from build123d import *

# Parameters (mm, degrees)
BOSS_EXTRUDE1_DEPTH            = 25
CUT_EXTRUDE1_REACH             = 60.44
SKETCH2_R                      = 2.25
SKETCH3_W                      = 25
SKETCH3_H                      = 63
SKETCH3_R                      = 3.75
BOSS_EXTRUDE2_DEPTH            = 2
FILLET1_R                      = 3
SKETCH4_R                      = 2.55
CUT_EXTRUDE2_DEPTH             = 3.5
SKETCH4_3_R                    = 2.55
CUT_EXTRUDE5_DEPTH             = 6.5
SKETCH6_W                      = 10
SKETCH6_H                      = 1.25
SKETCH5_R                      = 1.5
CUT_EXTRUDE3_DEPTH             = 1
SKETCH5_2_R                    = 1.5
CUT_EXTRUDE4_DEPTH             = 3.75
CUT_EXTRUDE4_DIRECTION_2_REACH = 59.567
CUT_EXTRUDE6_DEPTH             = 10


with BuildPart() as part:
    # Sketch1 → Boss-Extrude1 (new body)
    with BuildSketch(Plane(origin=(0, 0, 0), x_dir=(0, 0, -1), z_dir=(1, 0, 0))):
        Polygon((8.75, 0), (8.75, 9.25), (9.5, 10), (15.25, 10), (15.25, 23), (-19.25, 23), (-19.25, -40), (-16.25, -40), (-16.25, 0), (-12.5, 0), (-12.5, 8.25), (0, 8.25), (0, 0), (3.75, 0), align=None)
    extrude(amount=BOSS_EXTRUDE1_DEPTH)

    # Sketch2 → Cut-Extrude1 (cut, up to next)
    with BuildSketch(Plane.XY.offset(19.25), mode=Mode.PRIVATE) as cut_extrude1_sk1:
        with Locations((6.25, -30)):
            Circle(SKETCH2_R)
    cut_extrude1_tool1 = extrude(cut_extrude1_sk1.sketch, amount=-CUT_EXTRUDE1_REACH, mode=Mode.PRIVATE) & part.part
    # Sketch2 → Cut-Extrude1 (cut, up to next)
    with BuildSketch(Plane.XY.offset(19.25), mode=Mode.PRIVATE) as cut_extrude1_sk2:
        with Locations((6.25, -10)):
            Circle(SKETCH2_R)
    cut_extrude1_tool2 = extrude(cut_extrude1_sk2.sketch, amount=-CUT_EXTRUDE1_REACH, mode=Mode.PRIVATE) & part.part
    # Sketch2 → Cut-Extrude1 (cut, up to next)
    with BuildSketch(Plane.XY.offset(19.25), mode=Mode.PRIVATE) as cut_extrude1_sk3:
        with Locations((6.25, 16)):
            Circle(SKETCH2_R)
    cut_extrude1_tool3 = extrude(cut_extrude1_sk3.sketch, amount=-CUT_EXTRUDE1_REACH, mode=Mode.PRIVATE) & part.part
    # Sketch2 → Cut-Extrude1 (cut, up to next)
    with BuildSketch(Plane.XY.offset(19.25), mode=Mode.PRIVATE) as cut_extrude1_sk4:
        with Locations((19, 16)):
            Circle(SKETCH2_R)
    cut_extrude1_tool4 = extrude(cut_extrude1_sk4.sketch, amount=-CUT_EXTRUDE1_REACH, mode=Mode.PRIVATE) & part.part
    add(cut_extrude1_tool1.solids().sort_by_distance((6.25, -30, 19.25))[0], mode=Mode.SUBTRACT)
    add(cut_extrude1_tool2.solids().sort_by_distance((6.25, -10, 19.25))[0], mode=Mode.SUBTRACT)
    add(cut_extrude1_tool3.solids().sort_by_distance((6.25, 16, 19.25))[0], mode=Mode.SUBTRACT)
    add(cut_extrude1_tool4.solids().sort_by_distance((19, 16, 19.25))[0], mode=Mode.SUBTRACT)

    # Sketch3 → Boss-Extrude2 (add)
    with BuildSketch(Plane.XY.offset(19.25)):
        with Locations((12.5, -8.5)):
            Rectangle(SKETCH3_W, SKETCH3_H)
        with Locations((6.25, -30)):
            Circle(SKETCH3_R, mode=Mode.SUBTRACT)
        with Locations((6.25, -10)):
            Circle(SKETCH3_R, mode=Mode.SUBTRACT)
        Polygon((10, 18.165063509), (6.25, 20.330127019), (2.5, 18.165063509), (2.5, 13.834936491), (6.25, 11.669872981), (10, 13.834936491), align=None, mode=Mode.SUBTRACT)
        Polygon((19, 20.330127019), (15.25, 18.165063509), (15.25, 13.834936491), (19, 11.669872981), (22.75, 13.834936491), (22.75, 18.165063509), align=None, mode=Mode.SUBTRACT)
    extrude(amount=BOSS_EXTRUDE2_DEPTH)

    # Fillet1
    # the kernel refuses this fillet: 3 mm, written as the material it takes off along each edge
    with BuildSketch(Plane(origin=(3, 20, 18.25), x_dir=(0, 0, 1), z_dir=(-1, 0, 0))) as fillet1_piece_1_section:
        Polygon((0, 0), (FILLET1_R, 0), (FILLET1_R, FILLET1_R), (0, FILLET1_R), align=None)
    fillet1_piece_1 = extrude(amount=FILLET1_R, mode=Mode.PRIVATE)
    fillet1_piece_1 = fillet1_piece_1 - Plane(origin=(3, 20, 18.25), x_dir=(0, -0.7071067811865475, -0.7071067811865475), z_dir=(-1, 0, 0)) * Sphere(FILLET1_R, mode=Mode.PRIVATE)
    add(fillet1_piece_1, mode=Mode.SUBTRACT)
    with BuildSketch(Plane(origin=(22, 20, 18.25), x_dir=(0, 0, 1), z_dir=(1, 0, 0))) as fillet1_piece_2_section:
        Polygon((0, 0), (FILLET1_R, 0), (FILLET1_R, -FILLET1_R), (0, -FILLET1_R), align=None)
    fillet1_piece_2 = extrude(amount=FILLET1_R, mode=Mode.PRIVATE)
    fillet1_piece_2 = fillet1_piece_2 - Plane(origin=(22, 20, 18.25), x_dir=(0, -0.7071067811865475, -0.7071067811865475), z_dir=(1, 0, 0)) * Sphere(FILLET1_R, mode=Mode.PRIVATE)
    add(fillet1_piece_2, mode=Mode.SUBTRACT)
    with BuildSketch(Plane(origin=(0, 23, 18.25), x_dir=(1, 0, 0), z_dir=(0, 0, -1))) as fillet1_piece_3:
        with BuildLine():
            CenterArc((FILLET1_R, FILLET1_R), FILLET1_R, 180, 90)
            Line((0, FILLET1_R), (0, 0))
            Line((0, 0), (FILLET1_R, 0))
        make_face()
    extrude(amount=41, mode=Mode.SUBTRACT)
    with BuildSketch(Plane(origin=(25, 23, -22.75), x_dir=(0, -1, 0), z_dir=(0, 0, 1))) as fillet1_piece_4:
        with BuildLine():
            CenterArc((FILLET1_R, -FILLET1_R), FILLET1_R, 90, 90)
            Line((0, -FILLET1_R), (0, 0))
            Line((0, 0), (FILLET1_R, 0))
        make_face()
    extrude(amount=41, mode=Mode.SUBTRACT)
    with BuildSketch(Plane(origin=(22, 23, 21.25), x_dir=(0, -1, 0), z_dir=(-1, 0, 0))) as fillet1_piece_5:
        with BuildLine():
            CenterArc((FILLET1_R, -FILLET1_R), FILLET1_R, 90, 90)
            Line((0, -FILLET1_R), (0, 0))
            Line((0, 0), (FILLET1_R, 0))
        make_face()
    extrude(amount=19, mode=Mode.SUBTRACT)
    with BuildSketch(Plane(origin=(25, -47.5, 21.25), x_dir=(0, 0, -1), z_dir=(0, 1, 0))) as fillet1_piece_6:
        with BuildLine():
            CenterArc((FILLET1_R, FILLET1_R), FILLET1_R, 180, 90)
            Line((0, FILLET1_R), (0, 0))
            Line((0, 0), (FILLET1_R, 0))
        make_face()
    extrude(amount=67.5, mode=Mode.SUBTRACT)
    with BuildSketch(Plane(origin=(0, 20, 21.25), x_dir=(1, 0, 0), z_dir=(0, -1, 0))) as fillet1_piece_7:
        with BuildLine():
            CenterArc((FILLET1_R, -FILLET1_R), FILLET1_R, 90, 90)
            Line((0, -FILLET1_R), (0, 0))
            Line((0, 0), (FILLET1_R, 0))
        make_face()
    extrude(amount=67.5, mode=Mode.SUBTRACT)

    # Sketch4 → Cut-Extrude2 (cut)
    with BuildSketch(Plane.XY.offset(21.25)):
        Polygon((15.75, -12), (25, -12), (25, 8.5), (15.75, 8.5), (15.75, 7.65), (10, 7.65), (10, -3.15), (15.75, -3.15), align=None)
        with Locations((18.5, 3)):
            Circle(SKETCH4_R, mode=Mode.SUBTRACT)
    extrude(amount=-CUT_EXTRUDE2_DEPTH, mode=Mode.SUBTRACT)

    # Sketch4<3> → Cut-Extrude5 (cut)
    with BuildSketch(Plane.XY.offset(21.25)):
        with Locations((18.5, 3)):
            Circle(SKETCH4_3_R)
    extrude(amount=-CUT_EXTRUDE5_DEPTH, mode=Mode.SUBTRACT)

    # Sketch6 → Cut-Revolve1 (revolve, cut)
    with BuildSketch(Plane.XY.offset(21.25)):
        with Locations((5, 2.875)):
            Rectangle(SKETCH6_W, SKETCH6_H)
    revolve(axis=Axis((10, 2.25, 21.25), (-1, 0, 0)), mode=Mode.SUBTRACT)

    # Sketch5 → Cut-Extrude3 (cut, symmetric)
    with BuildSketch(Plane.XY.offset(17.75)):
        Polygon((1, 5.169872981), (6.5, 5.169872981), (6.5, 10.669872981), (1, 10.669872981), (0, 10.669872981), (0, 5.169872981), align=None)
        with Locations((3.75, 7.919872981)):
            Circle(SKETCH5_R, mode=Mode.SUBTRACT)
    extrude(amount=CUT_EXTRUDE3_DEPTH, both=True, mode=Mode.SUBTRACT)

    # Sketch5<2> → Cut-Extrude4 (cut)
    with BuildSketch(Plane.XY.offset(17.75)):
        with Locations(Location((3.75, 7.919872981, 0), (0, 0, 180))):
            Circle(SKETCH5_2_R)
    extrude(amount=-CUT_EXTRUDE4_DEPTH, mode=Mode.SUBTRACT)

    # Sketch5<2> → Cut-Extrude4 direction 2 (cut, up to next)
    with BuildSketch(Plane.XY.offset(17.75), mode=Mode.PRIVATE) as cut_extrude4_direction_2_sk1:
        with Locations(Location((3.75, 7.919872981, 0), (0, 0, 180))):
            Circle(SKETCH5_2_R)
    cut_extrude4_direction_2_tool1 = extrude(cut_extrude4_direction_2_sk1.sketch, amount=CUT_EXTRUDE4_DIRECTION_2_REACH, mode=Mode.PRIVATE) & part.part
    add(cut_extrude4_direction_2_tool1.solids().sort_by_distance((3.75, 7.919873, 17.75))[0], mode=Mode.SUBTRACT)

    # Sketch7 → Cut-Extrude6 (cut)
    with BuildSketch(Plane.XY.offset(19.25)):
        Polygon((22.75, 13.834936491), (22.75, 18.165063509), (19, 20.330127019), (15.25, 18.165063509), (15.25, 13.834936491), (19, 11.669872981), align=None)
        Polygon((6.25, 11.669872981), (10, 13.834936491), (10, 18.165063509), (6.25, 20.330127019), (2.5, 18.165063509), (2.5, 13.834936491), align=None)
    extrude(amount=-CUT_EXTRUDE6_DEPTH, mode=Mode.SUBTRACT)


solid = part.part
Here's how the part is built. I have some questions about the finished solid (model axes, mm). A direction names the side the tool comes from. Coordinates: 2 decimals unless noted, no trailing zeros. Loops run counter-clockwise (first coordinate to the right, second up) from the corner with the lowest first, then second, coordinate; pieces in that order, holes last.
1. Imagine slicing it at D-D, the plane x = 13.75. Please give me the cut outline in (y, z).
2. Imagine slicing it at C-C, the plane y = 16. Please give me the cut outline in (x, z).
3. For P1, Ø1, axis at x = 7.5, z = 15.5, coming from the -Y side; P2, Ø1.5, axis at x = 3, y = 7.5, coming from the +Z side; P3, Ø4, axis at x = 7.5, y = -9, coming from the +Z side, each with a flat end and sliding along its axis, tell me the tip position at first contact or that it passes through.
4. Imagine slicing it at B-B, the plane z = 2. Please give me the cut outline in (x, y), and give its area (3 significant figures).
5. For faces 4 (the flat face through (12, 0, 14)), 5 (the flat face through (10, 2.3, 19.5)), 6 (the cylindrical face through (3.945, 6.433, 19.982)), 7 (the cylindrical face through (5.3, 2.3, 20)), which set-ups out of +Z, -Z, +X, -X, +Y, -Y let a thin tool reach every point of the face, with its end or its side?
6. If we mould it in two halves opening along Z, with no side actions, what happens to faces 1 (the flat face through (4.349, 12.768, 15.166)), 2 (the flat face through (12, 16, -15.25)), 3 (the flat face through (12, 4, 0))? For each: pulls with the +Z half, pulls with the -Z half, needs draft (parallel to the pull), parting line crosses it, or undercut.
7. Imagine slicing it at A-A, the plane y = -30. Please give me the cut outline in (x, z).
8. I need wall thicknesses on L1, parallel to Z at x = 11.5, y = 1.5; L2, parallel to Y at x = 3.75, z = 15.6; L3, parallel to Y at x = 3.75, z = 20.55. Which ranges of each line are inside material? Lowest first, please.
Taken from the geometry:
1. outline: (-40, 16.25) - (0, 16.25) - (0, 12.5) - (8.25, 12.5) - (8.25, 0) - (0, 0) - (0, -8.75) - (9.25, -8.75) - (10, -9.5) - (10, -15.25) - (23, -15.25) - (23, 18.25) arc R3 ccw to (20, 21.25) - (7.65, 21.25) - (7.65, 17.75) - (-3.15, 17.75) - (-3.15, 21.25) - (-40, 21.25) - close
2. outline: (0, -15.25) - (4, -15.25) - (4, 9.25) - (2.5, 9.25) - (2.5, 21.21) arc R3 ccw to (0, 18.25) - close; (8.5, -15.25) - (16.75, -15.25) - (16.75, 9.25) - (15.25, 9.25) - (15.25, 21.25) - (10, 21.25) - (10, 9.25) - (8.5, 9.25) - close; (21.25, -15.25) - (25, -15.25) - (25, 18.25) arc R3 ccw to (22.75, 21.15) - (22.75, 9.25) - (21.25, 9.25) - close
3. P1: stops at y = 0
3. P2: stops at z = 21.24
3. P3: stops at z = 19.25
4. outline: (0, 8.25) - (25, 8.25) - (25, 20) arc R3 ccw to (22, 23) - (3, 23) arc R3 ccw to (0, 20) - close; hole circle Ø4.5 at (6.25, 16); hole circle Ø4.5 at (19, 16)
4. area: 333 mm2
5. face 4: -Z, +X, -X, -Y
5. face 5: +Z, +X
5. face 6: +Z
5. face 7: +Z, +X, -X
6. face 1: needs draft
6. face 2: pulls with the -Z half
6. face 3: undercut
7. outline: (0, 16.25) - (4, 16.25) - (4, 19.25) - (2.5, 19.25) - (2.5, 21.21) arc R3 ccw to (0, 18.25) - close; (8.5, 16.25) - (25, 16.25) - (25, 18.25) arc R3 ccw to (22, 21.25) - (10, 21.25) - (10, 19.25) - (8.5, 19.25) - close
8. L1: z = -8.75 to 0, 12.5 to 17.75
8. L2: y = 0 to 6.42, 9.42 to 13.11, 18.89 to 23
8. L3: y = -40 to -32.8, -27.2 to -12.8, -7.2 to 1.21, 3.29 to 6.42, 9.42 to 13.11, 18.89 to 21.93
